from build123d import *

# Parameters (mm, degrees)
SKETCH1_W                  = 50
SKETCH1_H                  = 10.2
BOSS_EXTRUDE1_DEPTH        = 6.25
F_4_0_4_DIAMETER_HOLE1_D   = 4
F_2_5_2_5_DIAMETER_HOLE1_D = 2.5
SKETCH6_W                  = 2
SKETCH6_H                  = 0.7
CUT_EXTRUDE1_DEPTH         = 51


with BuildPart() as part:
    # Sketch1 → Boss-Extrude1 (new body)
    with BuildSketch(Plane(origin=(0, 0, 0), x_dir=(1, 0, 0), z_dir=(0, 1, 0))):
        with Locations((25, 5.1)):
            Rectangle(SKETCH1_W, SKETCH1_H)
    extrude(amount=BOSS_EXTRUDE1_DEPTH)

    # Ø4.0 (4) Diameter Hole1 (through all)
    with Locations(Plane.XY):
        with Locations((4.75, 3.125), (45.25, 3.125)):
            Hole(F_4_0_4_DIAMETER_HOLE1_D / 2)

    # Ø2.5 (2.5) Diameter Hole1 (through all)
    with Locations(Plane(origin=(0, 6.25, 0), x_dir=(-1, 0, 0), z_dir=(0, 1, 0))):
        with Locations((-10, -5.1), (-40, -5.1)):
            Hole(F_2_5_2_5_DIAMETER_HOLE1_D / 2)

    # Sketch6 → Cut-Extrude1 (cut, through all)
    with BuildSketch(Plane(origin=(50, 0, 0), x_dir=(0, 0, -1), z_dir=(1, 0, 0))):
        with Locations((9.2, 0.35)):
            Rectangle(SKETCH6_W, SKETCH6_H)
    extrude(amount=-CUT_EXTRUDE1_DEPTH, mode=Mode.SUBTRACT)


solid = part.part
Input: part model. Units: mm. Frame: model coordinates. A direction names the side the tool comes from. Coordinates: 2 decimals unless noted, no trailing zeros. Order: outer loops, then holes, each group sorted by start corner. A loop starts at its lowest first (then second) coordinate and runs counter-clockwise, first axis right, second up. Notation, with made-up numbers: M 61,-24 L 100,-24 A26 cw 100,8 Z; hole C 27,47 d8. An arc over 180 degrees is marked long. Write item = value, one per line. Start each with the question number.
(1) Section B-B on z = -5.1. Output: boundary loops of the cut face in (x, y) (3 decimals), and give its area (3 significant figures).
(2) Section A-A on x = 45.25. Output: boundary loops of the cut face in (y, z) (3 decimals).
(3) First-contact query: P1, Ø1.6, axis at x = 12.5, z = -9.5, coming from the -Y side. Flat tip, straight axial feed; report the tip coordinate or a pass-through.
(4) Pull-direction query (X, two-part tool) for faces 3 (the cylindrical face through (38.75, 3.08, -5.05)), 4 (the flat face through (25, 0, -4)), 5 (the flat face through (50, 3, -5)); classes: released by +X, released by -X, zero draft, split by the parting line, or undercut.
(5) Section D-D on z = -0.5. Output: boundary loops of the cut face in (x, y) (3 decimals).
(6) Line query: line 1 along X through (y, z) = (3, -1); line 2 along Z through (x, y) = (40, 2.25); line 3 along Y through (x, z) = (45.25, -6.75) (3 decimals). Output: solid intervals per line, ascending. Write a range as [from, to].
(7) Section C-C on x = 30. Output: boundary loops of the cut face in (y, z), and give its area (4 significant figures).
(8) Reachability of faces 1 (the cylindrical face through (47.25, 3.21, -5.17)), 2 (the flat face through (25, 0.7, -9)) from +Z, -Z, +X, -X, +Y, -Y: full face, straight path, thin tool, end or side. Return the list, or none.
Result set:
q1.outline = M 0,0 L 8.75,0 L 8.75,6.25 L 0,6.25 Z; M 11.25,0 L 38.75,0 L 38.75,6.25 L 11.25,6.25 Z; M 41.25,0 L 50,0 L 50,6.25 L 41.25,6.25 Z; hole C 4.75,3.125 d4; hole C 45.25,3.125 d4
q1.area = 256 mm²
q2.outline = M 0,-8.2 L 0.7,-8.2 L 0.7,-10.2 L 1.125,-10.2 L 1.125,0 L 0,0 Z; M 5.125,-10.2 L 6.25,-10.2 L 6.25,0 L 5.125,0 Z
q3.P1 = 0.7
q4.face_3 = undercut
q4.face_4 = zero draft
q4.face_5 = released by +X
q5.outline = M 0,0 L 50,0 L 50,6.25 L 0,6.25 Z; hole C 4.75,3.125 d4; hole C 45.25,3.125 d4
q6.line_1 = [0, 2.75], [6.75, 43.25], [47.25, 50]
q6.line_2 = [-10.2, -6.35], [-3.85, 0]
q6.line_3 = [0, 1.125], [5.125, 6.25]
q7.outline = M 0,-8.2 L 0.7,-8.2 L 0.7,-10.2 L 6.25,-10.2 L 6.25,0 L 0,0 Z
q7.area = 62.35 mm²
q8.face_1 = +Z, -Z
q8.face_2 = -Z, +X, -X, -Y
